Input: dimensioned drawing with shaded views. Units: mm. Origin: part minimum x, y, z. A direction names the side the tool comes from. Give positions to 0.01 mm unless a question says otherwise; leave off trailing zeros. Order: outer loops, then holes, each group sorted by start corner. A loop starts at its lowest first (then second) coordinate and runs counter-clockwise, first axis right, second up. Notation, with made-up numbers: (84, 75.25) -> (107, 75.25) arc R33 cw to (107, 106.25) -> close; hole circle Ø2 at (10.5, 45). An arc over 180 degrees is marked (long way). Use CSV: the item, a comma, the result in double quotes.
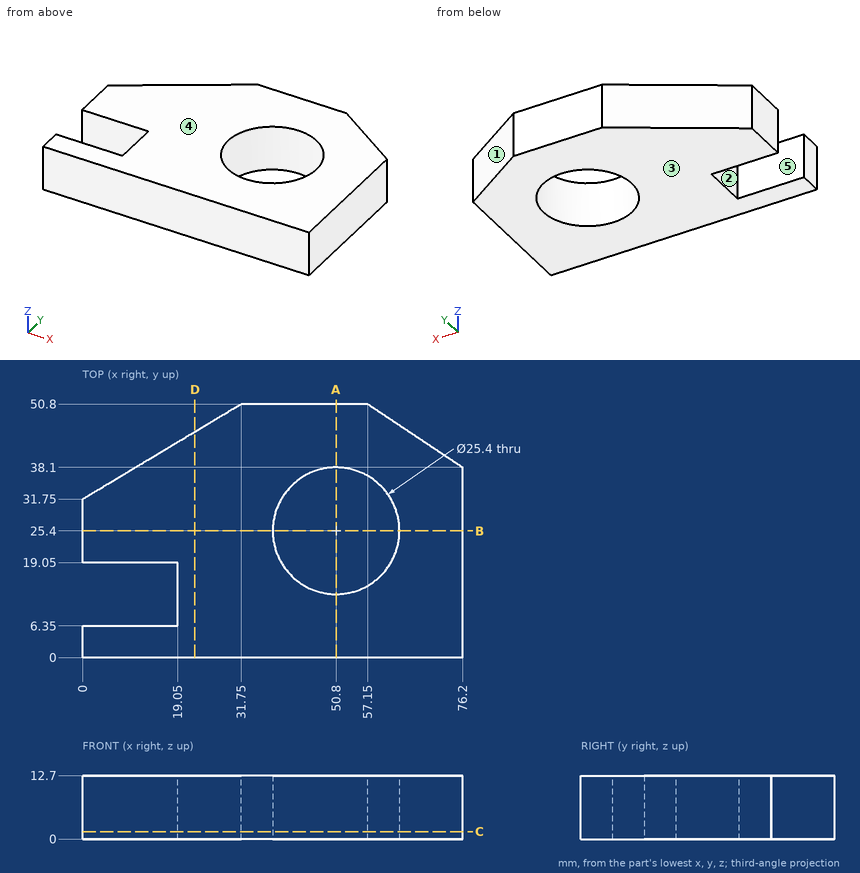
1. Pin query (flat end, axial travel): P1, Ø1, axis at y = 39, z = 9, coming from the -X side; P2, Ø6, axis at y = 39, z = 9.5, coming from the -X side. Return the tip coordinate at first contact, or that it passes through.
Answer below:
P1,"stops at x = 11.25"
P2,"stops at x = 7.08"
2. Section query A-A on x = 50.8. Return loops of the section in (y, z), plus the area to 3 significant figures.
Answer below:
outline,"(0, 0) -> (12.7, 0) -> (12.7, 12.7) -> (0, 12.7) -> close; (38.1, 0) -> (50.8, 0) -> (50.8, 12.7) -> (38.1, 12.7) -> close"
area,"323 mm²"
3. Section query B-B on y = 25.4. Return loops of the section in (x, z), plus the area to 3 significant figures.
Answer below:
outline,"(0, 0) -> (38.1, 0) -> (38.1, 12.7) -> (0, 12.7) -> close; (63.5, 0) -> (76.2, 0) -> (76.2, 12.7) -> (63.5, 12.7) -> close"
area,"645 mm²"
4. Mould query, pull axis Y, two halves, no side actions, for the marked faces 1, 2 and 3. Classes: released by +Y, released by -Y, zero draft, split by the parting line, or undercut.
Answer below:
face 1,"released by +Y"
face 2,"undercut"
face 3,"zero draft"
5. Section query D-D on x = 22.5. Return loops of the section in (y, z).
Answer below:
outline,"(0, 0) -> (45.25, 0) -> (45.25, 12.7) -> (0, 12.7) -> close"
6. Section query C-C on z = 1.5. Return loops of the section in (x, y).
Answer below:
outline,"(0, 0) -> (76.2, 0) -> (76.2, 38.1) -> (57.15, 50.8) -> (31.75, 50.8) -> (0, 31.75) -> (0, 19.05) -> (19.05, 19.05) -> (19.05, 6.35) -> (0, 6.35) -> close; hole circle Ø25.4 at (50.8, 25.4)"
7. Access query for the marked faces 4 and 5. Directions: +Z, -Z, +X, -X, +Y, -Y. A direction counts if a zero-diameter tool reaches every point of the face in a straight line with its end or side. Return the directions, or none.
Answer below:
face 4,"+Z, +X, -X, +Y, -Y"
face 5,"+Z, -Z, -X"
8. Ray query, line 1 along Y through (x, z) = (50.8, 7.5); line 2 along Y through (x, z) = (52.5, 10); line 3 along X through (y, z) = (17, 1). Return the intervals inside material, ascending.
Answer below:
line 1,"y = 0 to 12.7, 38.1 to 50.8"
line 2,"y = 0 to 12.81, 37.99 to 50.8"
line 3,"x = 19.05 to 41.27, 60.33 to 76.2"
